```python
from build123d import *

# Parameters (mm, degrees)
SKETCH1_R                       = 6.35
BOSS_EXTRUDE1_DEPTH             = 1.4
SKETCH2_W                       = 4
SKETCH2_H                       = 12.7
CUT_EXTRUDE1_DEPTH              = 2.2
SKETCH3_W                       = 12.7
SKETCH3_H                       = 4
CUT_EXTRUDE2_DEPTH              = 2.2
BOSS_EXTRUDE2_REACH             = 11.246
SKETCH9_R                       = 3.633
SKETCH9_R_2                     = 1.7
BOSS_EXTRUDE2_DIRECTION_2_REACH = 11.246


with BuildPart() as part:
    # Sketch1 → Boss-Extrude1 (new, symmetric)
    with BuildSketch(Plane.XY):
        Circle(SKETCH1_R)
    extrude(amount=BOSS_EXTRUDE1_DEPTH, both=True)

    # Sketch2 → Cut-Extrude1 (cut)
    with BuildSketch(Plane.XY.offset(1.4)):
        Rectangle(SKETCH2_W, SKETCH2_H)
    extrude(amount=-CUT_EXTRUDE1_DEPTH, mode=Mode.SUBTRACT)

    # Sketch3 → Cut-Extrude2 (cut)
    with BuildSketch(Plane(origin=(0, 0, -1.4), x_dir=(-1, 0, 0), z_dir=(0, 0, -1))):
        Rectangle(SKETCH3_W, SKETCH3_H)
    extrude(amount=-CUT_EXTRUDE2_DEPTH, mode=Mode.SUBTRACT)

    # Boss-Extrude2: up to this face of the body (flat: up to its plane)
    boss_extrude2_end = Plane(part.part.faces().sort_by_distance((-3.803983963, 0, 1.4))[0])
    # Sketch9 → Boss-Extrude2 (add, up to the picked face)
    with BuildSketch(Plane.XY.offset(-0.8), mode=Mode.PRIVATE) as boss_extrude2_sk1:
        Circle(SKETCH9_R)
        Circle(SKETCH9_R_2, mode=Mode.SUBTRACT)
    boss_extrude2_tool1 = split(extrude(boss_extrude2_sk1.sketch, amount=BOSS_EXTRUDE2_REACH, mode=Mode.PRIVATE), bisect_by=boss_extrude2_end, keep=Keep.BOTH, mode=Mode.PRIVATE)
    add(boss_extrude2_tool1.solids().sort_by(Axis((-3.530243, 0, -0.8), (0, 0, 1)))[0])

    # Boss-Extrude2 direction 2: up to this face of the body (flat: up to its plane)
    boss_extrude2_direction_2_end = Plane(part.part.faces().sort_by_distance((0, 3.803983963, -1.4))[0])
    # Sketch9 → Boss-Extrude2 direction 2 (add, up to the picked face)
    with BuildSketch(Plane.XY.offset(-0.8), mode=Mode.PRIVATE) as boss_extrude2_direction_2_sk1:
        Circle(SKETCH9_R)
        Circle(SKETCH9_R_2, mode=Mode.SUBTRACT)
    boss_extrude2_direction_2_tool1 = split(extrude(boss_extrude2_direction_2_sk1.sketch, amount=-BOSS_EXTRUDE2_DIRECTION_2_REACH, mode=Mode.PRIVATE), bisect_by=boss_extrude2_direction_2_end, keep=Keep.BOTH, mode=Mode.PRIVATE)
    add(boss_extrude2_direction_2_tool1.solids().sort_by(Axis((-3.530243, 0, -0.8), (0, 0, -1)))[0])


solid = part.part
```
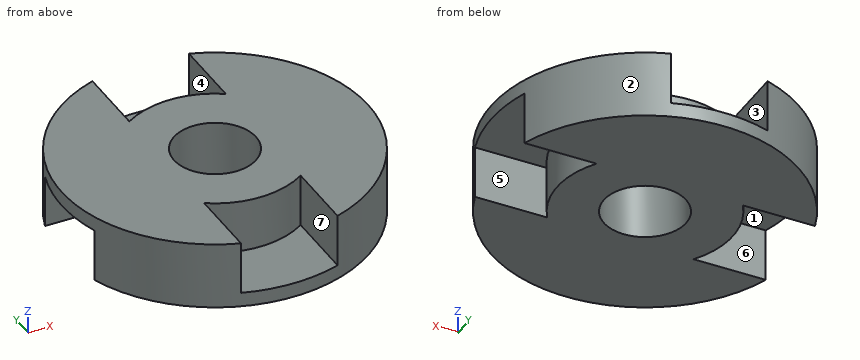
Read the model definition and answer for the solid it produces. Units are mm, in the model's axes. Face numbers are marked on the shaded views. A direction names the side the tool comes from. Round coordinates to 2 decimals unless told otherwise and drop trailing zeros. Loops run counter-clockwise (first coordinate to the right, second up) from the corner with the lowest first, then second, coordinate; pieces in that order, holes last. Notation, with made-up numbers: (47, -11.75) -> (61, -11.75) arc R18 ccw to (61, -5.75) -> close; hole circle Ø2 at (40.5, -36.75). An arc over 180 degrees is marked (long way). One line per item, written item: value.
1) Consider L1, parallel to X at y = 0, z = -0.25; L2, parallel to Z at x = 1, y = -5.5. Determine where each line is inside the solid, lowest interval first. Write a range as [from, to].
Answer list:
L1: x = [-3.63, -1.7], [1.7, 3.63]
L2: z = [-1.4, -0.8]
2) A cutting plane is placed at D-D (x = 5.5). Determine the outline of the cut face in (y, z), and give its area (3 significant figures).
Answer list:
outline: (-3.17, -1.4) -> (-2, -1.4) -> (-2, 0.8) -> (2, 0.8) -> (2, -1.4) -> (3.17, -1.4) -> (3.17, 1.4) -> (-3.17, 1.4) -> close
area: 8.97 mm²
3) The mould has two halves that part along X. Classify the marked faces 1, 2 and 3: pulls with the +X half, pulls with the -X half, needs draft (parallel to the pull), parting line crosses it, or undercut.
Answer list:
face 1: needs draft
face 2: parting line crosses it
face 3: undercut
4) Flat-ended cylindrical pins translate along their axes: P1, Ø1.5, axis at x = -3.5, z = 0, coming from the -Y side; P2, Ø0.7, axis at y = 5, z = 0.5, coming from the +X side; P3, Ø0.7, axis at x = 5, z = 0, coming from the -Y side. Find the tip coordinate at first contact, or state that the pin passes through.
Answer list:
P1: stops at y = -5.72
P2: stops at x = 4.32
P3: stops at y = -4.32
5) A cutting plane is placed at A-A (y = 0). Determine the outline of the cut face in (x, z), and give its area (3 significant figures).
Answer list:
outline: (-6.35, 0.8) -> (-3.63, 0.8) -> (-3.63, -1.4) -> (-1.7, -1.4) -> (-1.7, 1.4) -> (-6.35, 1.4) -> close; (1.7, -1.4) -> (3.63, -1.4) -> (3.63, 0.8) -> (6.35, 0.8) -> (6.35, 1.4) -> (1.7, 1.4) -> close
area: 14.1 mm²
6) For the marked faces 4, 5, 6 and 7, determine the directions among +Z, -Z, +X, -X, +Y, -Y from which every point of the face is accessible in a straight line to the end or side of a thin tool.
Answer list:
face 4: +Z, +Y
face 5: -Z, +X
face 6: -Z, -X
face 7: +Z, -Y
7) A cutting plane is placed at B-B (x = 0). Determine the outline of the cut face in (y, z).
Answer list:
outline: (-6.35, -1.4) -> (-1.7, -1.4) -> (-1.7, 1.4) -> (-3.63, 1.4) -> (-3.63, -0.8) -> (-6.35, -0.8) -> close; (1.7, -1.4) -> (6.35, -1.4) -> (6.35, -0.8) -> (3.63, -0.8) -> (3.63, 1.4) -> (1.7, 1.4) -> close
8) A cutting plane is placed at C-C (z = -1.05). Determine the outline of the cut face in (x, y).
Answer list:
outline: (-6.03, -2) arc R6.35 ccw to (6.03, -2) -> (3.03, -2) arc R3.63 ccw to (3.03, 2) -> (6.03, 2) arc R6.35 ccw to (-6.03, 2) -> (-3.03, 2) arc R3.63 ccw to (-3.03, -2) -> close; hole circle Ø3.4 at (0, 0)
